```python
from build123d import *


with BuildPart() as part:
    # Esquisse1 → Base-Révolution (revolve)
    with BuildSketch(Plane.XY, mode=Mode.PRIVATE) as base_r_volution_sk:
        Polygon((4, 0), (4.5, 0), (5, 0.5), (5, 10), (8, 10), (8, 11.5), (4, 11.5), align=None)
    revolve(base_r_volution_sk.sketch.rotate(Axis((0, 0, 0), (0, 1, 0)), 90), axis=Axis((0, 0, 0), (0, 1, 0)))


solid = part.part
```
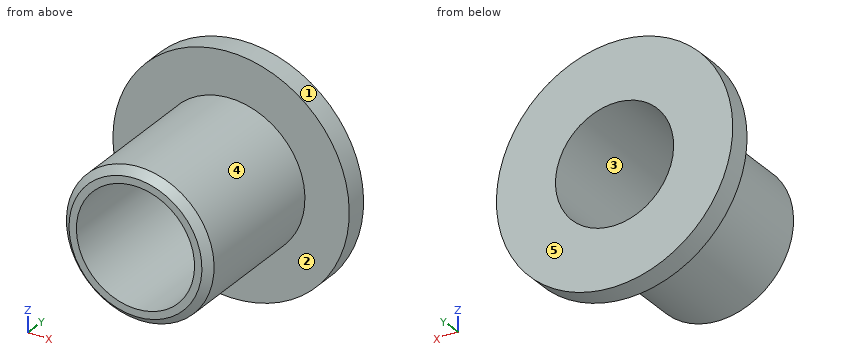
Work out the finished part from the listing and answer in its coordinate system (mm). Face numbers are marked on the shaded views. A direction names the side the tool comes from. Give positions to 0.01 mm unless a question says otherwise; leave off trailing zeros. Loops run counter-clockwise (first coordinate to the right, second up) from the corner with the lowest first, then second, coordinate; pieces in that order, holes last. Notation, with made-up numbers: (-9, 24.25) -> (20, 24.25) arc R15 ccw to (20, 53.25) -> close; hole circle Ø10 at (-3.5, 11). An arc over 180 degrees is marked (long way). Put each result on its own line as item: value. Start each with the question number.
Item 1: Find the intervals of material crossed by L1, parallel to X at y = 4.25, z = 0; L2, parallel to Y at x = -3.5, z = 4.5; L3, parallel to X at y = 5.75, z = 3.25, in increasing order. Write a range as [from, to].
Item 2: The part is cut by section A-A (z = 0). Give the vertices of the cut face in (x, y), then the cut area to 4 significant figures.
Item 3: Which of the six approach directions +Z, -Z, +X, -X, +Y, -Y give full straight-line access (tool end or side, diameter ignored) to the marked faces 4 and 5?
Item 4: The part is cut by section B-B (x = 0). Give the vertices of the cut face in (y, z).
Item 5: Each of these flat-tipped pins is pushed along its axis until it touches: P1, Ø1, axis at y = 10, z = 4, coming from the -X side; P2, Ø3, axis at x = -5, y = 3.5, coming from the -Z side; P3, Ø6, axis at x = -5.5, y = 10, coming from the -Z side; P4, Ø6.5, axis at x = 0, z = 0, coming from the -Y side. Where does it stop, or does it pass through?
Item 6: The part is cut by section C-C (y = 9.25). Give the vertices of the cut face in (x, z), then the cut area to 3 significant figures.
Item 7: The part is cut by section D-D (x = -6.25). Give the vertices of the cut face in (y, z).
Item 8: The mould has two halves that part along Z. Classify the marked faces 1, 2 and 3: released by +Z, released by -Z, zero draft, split by the parting line, or undercut.
Answers below:
1. L1: [-5, -4], [4, 5]
1. L2: [10, 11.5]
1. L3: [-3.8, -2.33], [2.33, 3.8]
2. outline: (-8, 10) -> (-5, 10) -> (-5, 0.5) -> (-4.5, 0) -> (-4, 0) -> (-4, 11.5) -> (-8, 11.5) -> close; (4, 0) -> (4.5, 0) -> (5, 0.5) -> (5, 10) -> (8, 10) -> (8, 11.5) -> (4, 11.5) -> close
2. area: 31.75 mm2
3. face 4: -Y
3. face 5: +Z, -Z, +X, -X, +Y
4. outline: (0, -4.5) -> (0.5, -5) -> (10, -5) -> (10, -8) -> (11.5, -8) -> (11.5, -4) -> (0, -4) -> close; (0, 4) -> (11.5, 4) -> (11.5, 8) -> (10, 8) -> (10, 5) -> (0.5, 5) -> (0, 4.5) -> close
5. P1: x = -7.19
5. P2: z = -3.57
5. P3: z = -7.6
5. P4: through
6. outline: circle Ø10 at (0, 0); hole circle Ø8 at (0, 0)
6. area: 28.3 mm2
7. outline: (10, -4.99) -> (11.5, -4.99) -> (11.5, 4.99) -> (10, 4.99) -> close
8. face 1: split by the parting line
8. face 2: zero draft
8. face 3: undercut
